Here's how the part is built. I have some questions about the finished solid (model axes, mm). Face numbers are marked on the shaded views. A direction names the side the tool comes from. Coordinates: 2 decimals unless noted, no trailing zeros. Write each loop counter-clockwise with the first axis right and the second up, starting at its lowest first coordinate (ties: lowest second). Pieces come first, ordered by that corner, then holes. Notation, with made-up numbers: M 10,-17 L 20,-17 A19 cw 20,-3 Z; hole C 54.25,77.25 d5. An arc over 180 degrees is marked long. Use one line per item in the form item = value. Start each with the question number.
1. Please list where these lines run through material, in increasing order: line 1 along Z through (x, y) = (-15, 0.15); line 2 along Z through (x, y) = (-11.5, 0.15); line 3 along Z through (x, y) = (-8, 0.8). Write a range as [from, to].
2. I want a section at B-B, the plane z = 3.75. List the corners of the cut face in (x, y) for me, plus the area to 3 significant figures.
3. I'm going to push flat-ended pins straight in: pin 1 Ø0.6 at (x, y) = (-16, 0.5) entering from +Z; pin 2 Ø0.7 at (y, z) = (0.5, 2) entering from +X; pin 3 Ø1 at (x, z) = (-16, 2.5) entering from -Y. Where does each tip first touch, or does it pass through?
4. Thinking about a two-plate mould opening in Z: for the marked faces 4, 5 and 6, which applies, released by +Z, released by -Z, zero draft, split by the parting line, or undercut?
5. I want a section at C-C, the plane y = 0.7. Count the separate pieces of the cut face and the enclosed holes in it, plus the area to 3 significant figures.
6. I want a section at D-D, the plane x = -6. List the corners of the cut face in (y, z) for me.
7. I want a section at A-A, the plane z = 5. List the corners of the cut face in (x, y) for me.
8. On a 3-axis mill with a long thin cutter (end or side, diameter ignored), from which of +Z, -Z, +X, -X, +Y, -Y can I reach the whole of each face in a straight line? I mean the marked faces 1, 2 and 3. Say none if no direction works.
from build123d import *

# Parameters (mm, degrees)
SKETCH1_R           = 1.397
BOSS_EXTRUDE1_DEPTH = 1.27
FILLET1_R           = 0.635
CUT_EXTRUDE3_DEPTH  = 2.286
CUT_EXTRUDE3_DRAFT  = -5


with BuildPart() as part:
    # Sketch1 → Boss-Extrude1 (new body)
    with BuildSketch(Plane(origin=(0, 0, 0), x_dir=(1, 0, 0), z_dir=(0, 1, 0))):
        with BuildLine():
            Line((0, 0), (-6.769261314, 0))
            Line((-6.769261314, 0), (-6.769261314, 3.81))
            Line((-6.769261314, 3.81), (-20.104261314, 3.81))
            ThreePointArc((-20.104261314, 3.81), (-26.839453405, 1.020192091), (-29.629261314, -5.715))
            Line((-29.629261314, -5.715), (-20.104261314, -2.17946963))
            Line((-20.104261314, -2.17946963), (-20.104261314, -0.90946963))
            Line((-20.104261314, -0.90946963), (-9.944261314, -0.90946963))
            ThreePointArc((-9.944261314, -0.90946963), (-7.404261314, -3.44946963), (-9.944261314, -5.98946963))
            Line((-9.944261314, -5.98946963), (-13.754261314, -5.98946963))
            ThreePointArc((-13.754261314, -5.98946963), (-12.534056747, -8.159663173), (-10.045804609, -8.244754297))
            ThreePointArc((-10.045804609, -8.244754297), (-5.162016489, -6.559807155), (0, -6.35))
            ThreePointArc((0, -6.35), (0.850738686, -3.175), (0, 0))
        make_face()
        with Locations((-1.689261314, -3.175)):
            Circle(SKETCH1_R, mode=Mode.SUBTRACT)
    extrude(amount=BOSS_EXTRUDE1_DEPTH)

    # Fillet1
    fillet1_edges = [part.edges().sort_by_distance(p)[0] for p in [
        (0, 0.635, 6.35),
        (-13.754261314, 0.635, 5.98946963),
        (-20.104261314, 0.635, 0.90946963),
        (-29.629261314, 0.635, 5.715),
        (-6.769261314, 0.635, -3.81),
        (0, 0.635, 0),
    ]]
    fillet(fillet1_edges, radius=FILLET1_R)


with BuildPart() as cut_extrude3_tool:
    # Sketch3 → Cut-Extrude3 (with draft: the straight prism first)
    with BuildSketch(Plane(origin=(0, 0.454734815, 0.454734815), x_dir=(1, 0, 0), z_dir=(0, 0.707106781, 0.707106781))):
        with BuildLine():
            ThreePointArc((-24.669594842, 2.353522249), (-18.89739116, 2.199678883), (-13.239594842, 3.353517673))
            Line((-13.239594842, 3.353517673), (-24.669594842, 2.353522249))
        make_face()
    extrude(amount=-CUT_EXTRUDE3_DEPTH)
    # Cut-Extrude3: the draft: its side faces are tilted about the plane it starts from
    cut_extrude3_sides = [cut_extrude3_tool.faces().sort_by_distance(p)[0] for p in [
        (-18.89739116, 1.201919619, -1.908896091),
        (-18.954594842, 1.664255078, -2.371231551),
    ]]
    draft(cut_extrude3_sides, Plane(origin=(0, 0.454734815, 0.454734815), x_dir=(1, 0, 0), z_dir=(0, 0.707106781, 0.707106781)), CUT_EXTRUDE3_DRAFT)


with BuildPart() as part_1:
    add(part.part)

    # Cut-Extrude3: cut by cut_extrude3_tool
    add(cut_extrude3_tool.part, mode=Mode.SUBTRACT)


solid = part_1.part
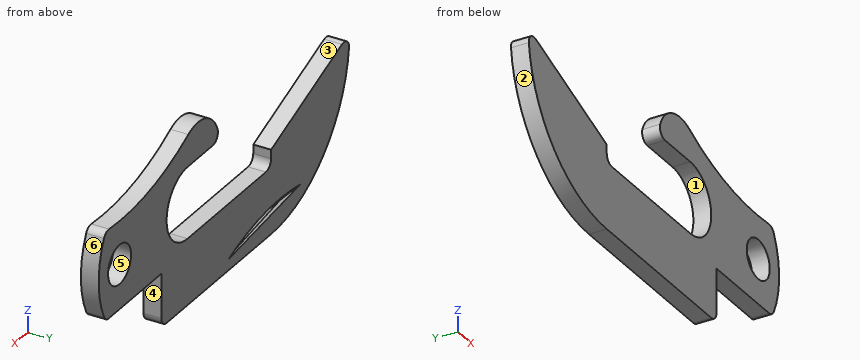
Answer list:
q1.line_1 = [-3.81, 0.91]
q1.line_2 = [-3.81, 0.91], [5.99, 8.51]
q1.line_3 = [-3.81, 1.82], [5.08, 7.34]
q2.outline = M -29.42,0 L -24.34,0 L -24.34,1.27 L -29.42,1.27 Z; M -7.42,0 L -2.96,0 L -2.96,1.27 L -7.42,1.27 Z; M -0.42,0 L 0.82,0 L 0.82,1.27 L -0.42,1.27 Z
q2.area = 13.7 mm²
q3.pin_1 = 0.91
q3.pin_2 = 0.8
q3.pin_3 = through
q4.face_4 = zero draft
q4.face_5 = undercut
q4.face_6 = split by the parting line
q5.separate_pieces = 1
q5.enclosed_holes = 2
q5.area = 175 mm²
q6.outline = M 0,0 L 1.27,0 L 1.27,6.74 L 0,6.74 Z
q7.outline = M -29.54,0 L -27.7,0 L -27.7,1.27 L -29.54,1.27 Z; M -7.93,0 L 0.58,0 L 0.58,1.27 L -7.93,1.27 Z
q8.face_1 = +Y, -Y
q8.face_2 = -Z, -X, +Y, -Y
q8.face_3 = +Z, +Y, -Y
